Can you work these out from the model? Positions are in its coordinate system, mm. Face numbers are marked on the shaded views. A direction names the side the tool comes from. Round coordinates to 2 decimals unless told otherwise and drop trailing zeros. Loops run counter-clockwise (first coordinate to the right, second up) from the corner with the lowest first, then second, coordinate; pieces in that order, holes last. Notation, with made-up numbers: (17, 54) -> (26, 54) arc R17 ccw to (26, 61) -> close; hole circle Ø4 at (-5.75, 34). An arc over 180 degrees is marked (long way). Answer as a JSON object with one key per item and string values.
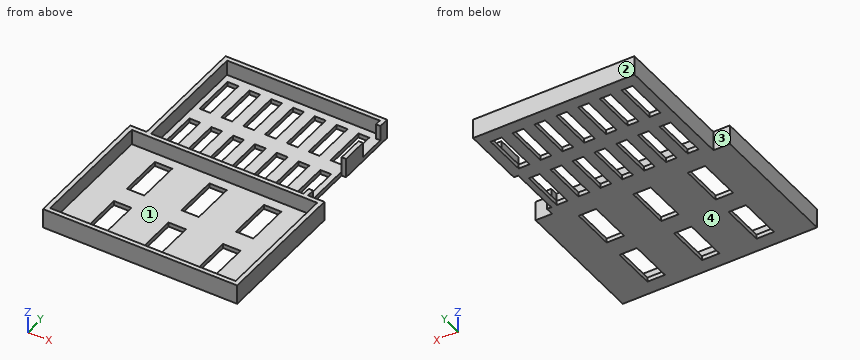
```python
from build123d import *

# Parameters (mm, degrees)
SKETCH1_W             = 5
SKETCH1_H             = 20
BOSS_EXTRUDE1_DEPTH   = 2
SKETCH1_W_2           = 8
BOSS_EXTRUDE1_2_DEPTH = 2
SKETCH1_3_W           = 85
SKETCH1_3_H           = 58.381043258
SKETCH1_3_W_2         = 2
SKETCH1_3_H_2         = 12
BOSS_EXTRUDE2_DEPTH   = 9


with BuildPart() as part:
    # Sketch1 → Boss-Extrude1 (new body)
    with BuildSketch(Plane.XY):
        Polygon((37, 12), (37, 24.5), (35, 24.5), (35, 27.25), (0, 27.25), (-35, 27.25), (-35, -27.25), (35, -27.25), (35, 12), align=None)
        with Locations((-30, -13.625)):
            Rectangle(SKETCH1_W, SKETCH1_H, mode=Mode.SUBTRACT)
        with Locations((-20, -13.625)):
            Rectangle(SKETCH1_W, SKETCH1_H, mode=Mode.SUBTRACT)
        with Locations((-10, -13.625)):
            Rectangle(SKETCH1_W, SKETCH1_H, mode=Mode.SUBTRACT)
        with Locations((0, -13.625)):
            Rectangle(SKETCH1_W, SKETCH1_H, mode=Mode.SUBTRACT)
        with Locations((10, -13.625)):
            Rectangle(SKETCH1_W, SKETCH1_H, mode=Mode.SUBTRACT)
        with Locations((20, -13.625)):
            Rectangle(SKETCH1_W, SKETCH1_H, mode=Mode.SUBTRACT)
        with Locations((30, -13.625)):
            Rectangle(SKETCH1_W, SKETCH1_H, mode=Mode.SUBTRACT)
        with Locations((-30, 13.625)):
            Rectangle(SKETCH1_W, SKETCH1_H, mode=Mode.SUBTRACT)
        with Locations((-20, 13.625)):
            Rectangle(SKETCH1_W, SKETCH1_H, mode=Mode.SUBTRACT)
        with Locations((-10, 13.625)):
            Rectangle(SKETCH1_W, SKETCH1_H, mode=Mode.SUBTRACT)
        Polygon((-2.5, 23.625), (0, 23.625), (2.5, 23.625), (2.5, 3.625), (0, 3.625), (-2.5, 3.625), align=None, mode=Mode.SUBTRACT)
        with Locations((10, 13.625)):
            Rectangle(SKETCH1_W, SKETCH1_H, mode=Mode.SUBTRACT)
        with Locations((20, 13.625)):
            Rectangle(SKETCH1_W, SKETCH1_H, mode=Mode.SUBTRACT)
        with Locations((30, 13.625)):
            Rectangle(SKETCH1_W, SKETCH1_H, mode=Mode.SUBTRACT)
    extrude(amount=BOSS_EXTRUDE1_DEPTH)



with BuildPart() as body_2:
    # Sketch1 → Boss-Extrude1 2 (new body)
    with BuildSketch(Plane.XY):
        Polygon((0, -29.25), (-42.5, -29.25), (-42.5, -87.631043258), (42.5, -87.631043258), (42.5, -29.25), align=None)
        with Locations((-25, -73.035782443)):
            Rectangle(SKETCH1_W_2, SKETCH1_H, mode=Mode.SUBTRACT)
        with Locations((0, -73.035782443)):
            Rectangle(SKETCH1_W_2, SKETCH1_H, mode=Mode.SUBTRACT)
        with Locations((-25, -43.845260814)):
            Rectangle(SKETCH1_W_2, SKETCH1_H, mode=Mode.SUBTRACT)
        Polygon((-4, -33.845260814), (0, -33.845260814), (4, -33.845260814), (4, -53.845260814), (0, -53.845260814), (-4, -53.845260814), align=None, mode=Mode.SUBTRACT)
        with Locations((25, -73.035782443)):
            Rectangle(SKETCH1_W_2, SKETCH1_H, mode=Mode.SUBTRACT)
        with Locations((25, -43.845260814)):
            Rectangle(SKETCH1_W_2, SKETCH1_H, mode=Mode.SUBTRACT)
    extrude(amount=BOSS_EXTRUDE1_2_DEPTH)


with BuildPart() as part_1:
    add(part.part)

    add(body_2.part)  # Boss-Extrude2 merges body 2
    # Sketch1<3> → Boss-Extrude2 (add)
    # profile 1 of 2: a face of its own
    with BuildSketch(Plane.XY):
        Polygon((37, 29.25), (-37, 29.25), (-37, -27.25), (-44.5, -27.25), (-44.5, -89.631043258), (44.5, -89.631043258), (44.5, -27.25), (37, -27.25), (37, -23.625), (35, -23.625), (35, -27.25), (-35, -27.25), (-35, 27.25), (35, 27.25), (35, 24.5), (37, 24.5), align=None)
        with Locations((0, -58.440521629)):
            Rectangle(SKETCH1_3_W, SKETCH1_3_H, mode=Mode.SUBTRACT)
    # profile 2 of 2: a face of its own
    with BuildSketch(Plane.XY):
        with Locations((36, 6)):
            Rectangle(SKETCH1_3_W_2, SKETCH1_3_H_2)
    extrude(amount=BOSS_EXTRUDE2_DEPTH)


solid = part_1.part
```
Q1. I want a section at A-A, the plane z = 6.5. Write out the boundary of the cut face in (x, y) (3 decimals).
Determined:
{"outline": "(-44.5, -89.631) -> (44.5, -89.631) -> (44.5, -27.25) -> (37, -27.25) -> (37, -23.625) -> (35, -23.625) -> (35, -27.25) -> (-35, -27.25) -> (-35, 27.25) -> (35, 27.25) -> (35, 24.5) -> (37, 24.5) -> (37, 29.25) -> (-37, 29.25) -> (-37, -27.25) -> (-44.5, -27.25) -> close; (35, 0) -> (37, 0) -> (37, 12) -> (35, 12) -> close; hole (-42.5, -87.631) -> (42.5, -87.631) -> (42.5, -29.25) -> (-42.5, -29.25) -> close"}
Q2. On a 3-axis mill with a long thin cutter (end or side, diameter ignored), from which of +Z, -Z, +X, -X, +Y, -Y can I reach the whole of each face in a straight line? I mean the marked faces 3 and 4. Say none if no direction works.
Determined:
{"face 3": "+Z, -Z, -X, +Y", "face 4": "-Z, +X, -X, +Y, -Y"}
Q3. I'm going to push flat-ended pins straight in: pin 1 (1 mm diameter, centred on y = -12, z = 1.5, fed in from +X); pin 2 (2 mm diameter, centred on y = 17.5, z = 0.5, fed in from +X); pin 3 (1 mm diameter, centred on y = -16.5, z = 1, fed in from -X). Where does each tip first touch, or does it pass through?
Determined:
{"pin 1": "x = 35", "pin 2": "x = 37", "pin 3": "x = -37"}
Q4. I want a section at C-C, the plane x = -26. Write out the boundary of the cut face in (y, z), then the cut area to 3 significant figures.
Determined:
{"outline": "(-89.63, 0) -> (-83.04, 0) -> (-83.04, 2) -> (-87.63, 2) -> (-87.63, 9) -> (-89.63, 9) -> close; (-63.04, 0) -> (-53.85, 0) -> (-53.85, 2) -> (-63.04, 2) -> close; (-33.85, 0) -> (29.25, 0) -> (29.25, 9) -> (27.25, 9) -> (27.25, 2) -> (-27.25, 2) -> (-27.25, 9) -> (-29.25, 9) -> (-29.25, 2) -> (-33.85, 2) -> close", "area": "200 mm²"}
Q5. We'd pull the mould along X, two halves only. Please class the marked faces 1 and 2: pulls with the +X half, pulls with the -X half, needs draft (parallel to the pull), parting line crosses it, or undercut.
Determined:
{"face 1": "undercut", "face 2": "needs draft"}
Q6. I want a section at B-B, the plane y = -10. Give the number of separate pieces and of enclosed holes in the cut face, then the cut area to 3 significant figures.
Determined:
{"separate pieces": "8", "enclosed holes": "0", "area": "88.0 mm²"}
Q7. I want a section at D-D, the plane y = -73. Write out the boundary of the cut face in (x, z), then the cut area to 3 significant figures.
Determined:
{"outline": "(-44.5, 0) -> (-29, 0) -> (-29, 2) -> (-42.5, 2) -> (-42.5, 9) -> (-44.5, 9) -> close; (-21, 0) -> (-4, 0) -> (-4, 2) -> (-21, 2) -> close; (4, 0) -> (21, 0) -> (21, 2) -> (4, 2) -> close; (29, 0) -> (44.5, 0) -> (44.5, 9) -> (42.5, 9) -> (42.5, 2) -> (29, 2) -> close", "area": "158 mm²"}
Q8. If I drill on L1, parallel to Y at x = 6, z = 8.25; L2, parallel to X at y = -65, z = 4.25, over which ranges is the centre line in solid material (lowest first)? Write a range as [from, to].
Determined:
{"L1": "[-89.63, -87.63], [-29.25, -27.25], [27.25, 29.25]", "L2": "[-44.5, -42.5], [42.5, 44.5]"}
